Work out the finished part from the listing and answer in its coordinate system (mm). Face numbers are marked on the shaded views. Round coordinates to 2 decimals unless told otherwise and drop trailing zeros. Order: outer loops, then holes, each group sorted by start corner. A loop starts at its lowest first (then second) coordinate and runs counter-clockwise, first axis right, second up. Notation, with made-up numbers: (-31, -1.5) -> (22, -1.5) arc R19 cw to (22, 12.5) -> close; hole circle Ø10 at (83.5, -31.5). An arc over 180 degrees is marked (long way). Use a Markdown table: item, result. Add a question column.
Item 1: Find the intervals of material crossed by L1, parallel to Z at x = -25, y = 1; L2, parallel to Y at x = -25.4, z = -45.75, in increasing order. Write a range as [from, to].
Item 2: For a pull along Y with two mould halves and no side action, classify the marked faces 1, 2 and 3 as +Y half, -Y half, draft (parallel to the pull), parting line (faces both ways), or undercut.
Item 3: Flat-ended cylindrical pins translate along their axes: P1, Ø9, axis at x = -25.4, z = -25.4, coming from the +Y side; P2, Ø8, axis at x = 25.4, y = 76.2, coming from the +Z side; P3, Ø6.5, axis at x = 25.4, y = 25.4, coming from the -Z side. Find the tip coordinate at first contact, or state that the pin passes through.
Item 4: A cutting plane is placed at C-C, the plane y = 76.2. Determine the outline of the cut face in (x, z), plus the area to 3 significant figures.
Item 5: A cutting plane is placed at B-B, the plane z = -25.4. Determine the outline of the cut face in (x, y).
Item 6: A cutting plane is placed at D-D, the plane x = 20. Determine the outline of the cut face in (y, z).
Item 7: A cutting plane is placed at A-A, the plane x = -25.4. Determine the outline of the cut face in (y, z).
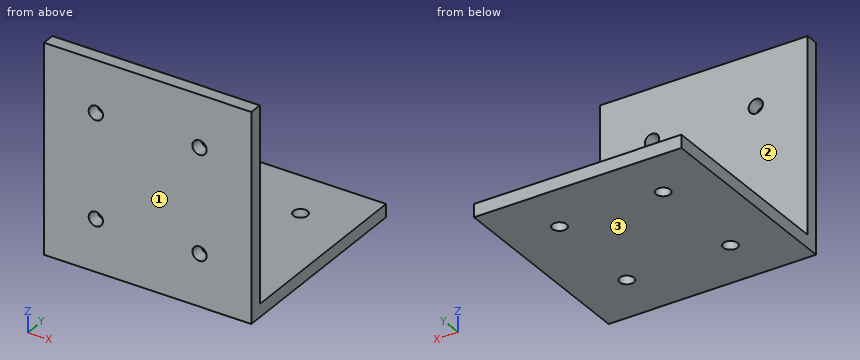
from build123d import *

# Parameters (mm, degrees)
SKETCH1_W           = 101.6
SKETCH1_H           = 101.6
SKETCH1_R           = 3.4925
BOSS_EXTRUDE1_DEPTH = 6.35
SKETCH2_W           = 101.6
SKETCH2_H           = 6.35
BOSS_EXTRUDE2_DEPTH = 95.25
SKETCH3_R           = 3.4925
CUT_EXTRUDE1_DEPTH  = 6.35


with BuildPart() as part:
    # Sketch1 → Boss-Extrude1 (new body)
    with BuildSketch(Plane(origin=(0, 0, 0), x_dir=(1, 0, 0), z_dir=(0, 1, 0))):
        Rectangle(SKETCH1_W, SKETCH1_H)
        with Locations(Location((-25.4, 25.4, 0), (0, 0, 270))):
            Circle(SKETCH1_R, mode=Mode.SUBTRACT)
        with Locations(Location((25.4, 25.4, 0), (0, 0, 270))):
            Circle(SKETCH1_R, mode=Mode.SUBTRACT)
        with Locations(Location((25.4, -25.4, 0), (0, 0, 270))):
            Circle(SKETCH1_R, mode=Mode.SUBTRACT)
        with Locations(Location((-25.4, -25.4, 0), (0, 0, 270))):
            Circle(SKETCH1_R, mode=Mode.SUBTRACT)
    extrude(amount=BOSS_EXTRUDE1_DEPTH)

    # Sketch2 → Boss-Extrude2 (add)
    with BuildSketch(Plane(origin=(0, 6.35, 0), x_dir=(1, 0, 0), z_dir=(0, 1, 0))):
        with Locations((0, 47.625)):
            Rectangle(SKETCH2_W, SKETCH2_H)
    extrude(amount=BOSS_EXTRUDE2_DEPTH)

    # Sketch3 → Cut-Extrude1 (cut)
    with BuildSketch(Plane(origin=(0, 0, -50.8), x_dir=(-1, 0, 0), z_dir=(0, 0, -1))):
        with Locations((-25.4, 76.2)):
            Circle(SKETCH3_R)
        with Locations((25.4, 76.2)):
            Circle(SKETCH3_R)
        with Locations((25.4, 25.4)):
            Circle(SKETCH3_R)
        with Locations((-25.4, 25.4)):
            Circle(SKETCH3_R)
    extrude(amount=-CUT_EXTRUDE1_DEPTH, mode=Mode.SUBTRACT)


solid = part.part
Reported:
| question | item | result |
|---|---|---|
| 1 | L1 | [-50.8, -28.87], [-21.93, 21.93], [28.87, 50.8] |
| 1 | L2 | [0, 21.91], [28.89, 72.71], [79.69, 101.6] |
| 2 | face 1 | -Y half |
| 2 | face 2 | +Y half |
| 2 | face 3 | draft |
| 3 | P1 | y = 6.35 |
| 3 | P2 | z = -44.45 |
| 3 | P3 | through |
| 4 | outline | (-50.8, -50.8) -> (-28.89, -50.8) -> (-28.89, -44.45) -> (-50.8, -44.45) -> close; (-21.91, -50.8) -> (21.91, -50.8) -> (21.91, -44.45) -> (-21.91, -44.45) -> close; (28.89, -50.8) -> (50.8, -50.8) -> (50.8, -44.45) -> (28.89, -44.45) -> close |
| 4 | area | 556 mm² |
| 5 | outline | (-50.8, 0) -> (-28.89, 0) -> (-28.89, 6.35) -> (-50.8, 6.35) -> close; (-21.91, 0) -> (21.91, 0) -> (21.91, 6.35) -> (-21.91, 6.35) -> close; (28.89, 0) -> (50.8, 0) -> (50.8, 6.35) -> (28.89, 6.35) -> close |
| 6 | outline | (0, -50.8) -> (101.6, -50.8) -> (101.6, -44.45) -> (6.35, -44.45) -> (6.35, 50.8) -> (0, 50.8) -> close |
| 7 | outline | (0, -50.8) -> (21.91, -50.8) -> (21.91, -44.45) -> (6.35, -44.45) -> (6.35, -28.89) -> (0, -28.89) -> close; (0, -21.91) -> (6.35, -21.91) -> (6.35, 21.91) -> (0, 21.91) -> close; (0, 28.89) -> (6.35, 28.89) -> (6.35, 50.8) -> (0, 50.8) -> close; (28.89, -50.8) -> (72.71, -50.8) -> (72.71, -44.45) -> (28.89, -44.45) -> close; (79.69, -50.8) -> (101.6, -50.8) -> (101.6, -44.45) -> (79.69, -44.45) -> close |
